from build123d import *

# Parameters (mm, degrees)
EXTRUDE_1_DEPTH     = 14
SKETCH_2_R          = 1.65
CUT_EXTRUDE_1_DEPTH = 2
SKETCH_3_R          = 1.4
CUT_EXTRUDE_2_DEPTH = 14
FILLET_1_R          = 3
SKETCH_5_R          = 0.6
SKETCH_5_R_2        = 1
CUT_EXTRUDE_3_DEPTH = 10


with BuildPart() as part:
    # 草图1 → 凸台-拉伸1 (new body)
    with BuildSketch(Plane.XY):
        Polygon((-28.25, 0), (-28.25, 19), (28.25, 19), (28.25, 0), (26.25, 0), (26.25, 16), (-26.25, 16), (-26.25, 0), align=None)
    extrude(amount=EXTRUDE_1_DEPTH)

    # 草图2 → 切除-拉伸1 (cut)
    with BuildSketch(Plane(origin=(28.25, 0, 0), x_dir=(0, 0, -1), z_dir=(1, 0, 0))):
        with Locations((-7, 5)):
            Circle(SKETCH_2_R)
    extrude(amount=-CUT_EXTRUDE_1_DEPTH, mode=Mode.SUBTRACT)

    # 草图3 → 切除-拉伸2 (cut)
    with BuildSketch(Plane(origin=(0, 19, 0), x_dir=(1, 0, 0), z_dir=(0, 1, 0))):
        with Locations((-18.98, -7)):
            Circle(SKETCH_3_R)
        with Locations((10.48, -7)):
            Circle(SKETCH_3_R)
    extrude(amount=-CUT_EXTRUDE_2_DEPTH, mode=Mode.SUBTRACT)

    # 圆角1
    fillet_1_edges = [part.edges().sort_by_distance(p)[0] for p in [
        (-27.25, 0, 0),
        (27.25, 0, 0),
        (27.25, 0, 14),
        (-27.25, 0, 14),
    ]]
    fillet(fillet_1_edges, radius=FILLET_1_R)

    # 草图5 → 切除-拉伸3 (cut)
    with BuildSketch(Plane.ZY.offset(28.25)):
        with Locations((7, 9.085)):
            Circle(SKETCH_5_R)
        with Locations((7, 13.085)):
            Circle(SKETCH_5_R)
        with Locations((7, 5)):
            Circle(SKETCH_5_R_2)
    extrude(amount=-CUT_EXTRUDE_3_DEPTH, mode=Mode.SUBTRACT)


solid = part.part
Here's how the part is built. I have some questions about the finished solid (model axes, mm). A direction names the side the tool comes from. Coordinates: 2 decimals unless noted, no trailing zeros. Loops run counter-clockwise (first coordinate to the right, second up) from the corner with the lowest first, then second, coordinate; pieces in that order, holes last. Notation, with made-up numbers: (-17.5, -5.75) -> (0.5, -5.75) arc R18 cw to (0.5, 16.25) -> close; hole circle Ø5 at (-32.75, 73.5). An arc over 180 degrees is marked (long way). Use one line per item in the form item = value. Start each with the question number.
(1) Please list where these lines run through material, in increasing order: line 1 along Y through (x, z) = (-27.75, 7) (3 decimals); line 2 along Z through (x, y) = (-18.98, 18.1); line 3 along X through (y, z) = (9, 8.5).
(2) If we section it at C-C (x = 10.48): Please give me the cut outline in (y, z).
(3) If we section it at D-D (y = 15): Please give me the cut outline in (x, z), then the cut area to 3 significant figures.
(4) Will these pins go through, and if not, where does the flat tip stop? pin 1 (1.7 mm diameter, centred on x = 10.48, z = 7, fed in from -Y); pin 2 (1.5 mm diameter, centred on x = -20, z = 10.5, fed in from -Y); pin 3 (3 mm diameter, centred on y = 5, z = 7, fed in from -X); pin 4 (1 mm diameter, centred on y = 13.085, z = 7, fed in from -X).
(5) If we section it at A-A (y = 5): Please give me the cut outline in (x, z).
(6) We'd pull the mould along Z, two halves only. Please class faces 1 (the face through (-27, 0, 7)), 2 (the face through (27.24, 0.9, 0.86)), 3 (the face through (-27.264, 5.676, 6.263)), 4 (the face through (-20.09, 17.52, 7.85)): pulls with the +Z half, pulls with the -Z half, needs draft (parallel to the pull), parting line crosses it, or undercut.
(7) If we section it at B-B (z = 7): Give the number of separate pieces and of enclosed holes in the cut face, then the cut area to 3 significant figures.
(8) On a 3-axis mill with a long thin cutter (end or side, diameter ignored), from which of +Z, -Z, +X, -X, +Y, -Y can I reach the whole of each face in a straight line? I mean faces 5 (the face through (-26.25, 8, 7)), 6 (the face through (-27.264, 13.591, 7.323)), 7 (the face through (27.26, 4, 8.31)), 8 (the face through (0, 19, 7)). Say none if no direction works.
Verdict:
q1.line_1 = 0 to 4, 6 to 8.485, 9.685 to 12.485, 13.685 to 19
q1.line_2 = 0 to 5.6, 8.4 to 14
q1.line_3 = -28.25 to -26.25, 26.25 to 28.25
q2.outline = (16, 0) -> (19, 0) -> (19, 5.6) -> (16, 5.6) -> close; (16, 8.4) -> (19, 8.4) -> (19, 14) -> (16, 14) -> close
q3.outline = (-28.25, 0) -> (-26.25, 0) -> (-26.25, 14) -> (-28.25, 14) -> close; (26.25, 0) -> (28.25, 0) -> (28.25, 14) -> (26.25, 14) -> close
q3.area = 56.0 mm²
q4.pin_1 = through
q4.pin_2 = 16
q4.pin_3 = -28.25
q4.pin_4 = 26.25
q5.outline = (-28.25, 0) -> (-26.25, 0) -> (-26.25, 6) -> (-28.25, 6) -> close; (-28.25, 8) -> (-26.25, 8) -> (-26.25, 14) -> (-28.25, 14) -> close; (26.25, 0) -> (28.25, 0) -> (28.25, 5.35) -> (26.25, 5.35) -> close; (26.25, 8.65) -> (28.25, 8.65) -> (28.25, 14) -> (26.25, 14) -> close
q6.face_1 = needs draft
q6.face_2 = pulls with the -Z half
q6.face_3 = undercut
q6.face_4 = undercut
q7.separate_pieces = 7
q7.enclosed_holes = 0
q7.area = 201 mm²
q8.face_5 = +Z, -Z, -Y
q8.face_6 = -X
q8.face_7 = +X
q8.face_8 = +Z, -Z, +X, -X, +Y
